Model file for the job. Use its own axes, mm. Give positions to 0.01 mm unless a question says otherwise; leave off trailing zeros. Order: outer loops, then holes, each group sorted by start corner. A loop starts at its lowest first (then second) coordinate and runs counter-clockwise, first axis right, second up. Notation, with made-up numbers: (-31.5, -11.75) -> (23.5, -11.75) arc R10 ccw to (23.5, -5.75) -> close; hole circle Ø10 at (19.5, 1.25). An arc over 180 degrees is marked (long way). Use CSV: the item, a comma, the result in double quotes. Start each with the question number.
1. Cut at C-C on z = -2. List the corners of the cut face in (x, y).
2. Cut at D-D on x = 61. List the corners of the cut face in (y, z) (3 decimals).
3. Cut at A-A on y = -50.8. List the corners of the cut face in (x, z) (3 decimals).
4. Wall check: line 1 (Y direction, x = 0, z = -1); line 2 (X direction, y = -52, z = -0.5); line 3 (X direction, y = -48.5, z = 0.25). Give the ranges that are in metal, low to high. Write a range as from..to.
5. Drop flat-ended pins along their axis: pin 1 (1 mm diameter, centred on y = -60.5, z = -1.5, fed in from -X); pin 2 (14.5 mm diameter, centred on x = 0, y = -50.8, fed in from -Z) (3 decimals); pin 3 (2 mm diameter, centred on x = 78.5, z = 2, fed in from -Y). Give the stop position or say it passes through.
6. Cut at B-B on x = 0. List the corners of the cut face in (y, z) (3 decimals), then the cut area to 3 significant figures.
```python
from build123d import *

# Parameters (mm, degrees)
BOSS_EXTRUDE1_DEPTH = 3.175
SKETCH2_R           = 6.35
CUT_EXTRUDE1_DEPTH  = 136.152108752


with BuildPart() as part:
    # Sketch1 → Boss-Extrude1 (new, symmetric)
    with BuildSketch(Plane.XY):
        Polygon((-101.6, 0), (-12.7, -88.9), (12.7, -88.9), (101.6, 0), align=None)
    extrude(amount=BOSS_EXTRUDE1_DEPTH, both=True)

    # Sketch2 → Cut-Extrude1 (cut, through all)
    with BuildSketch(Plane.XY.offset(3.175)):
        with Locations((0, -50.8)):
            Circle(SKETCH2_R)
    extrude(amount=-CUT_EXTRUDE1_DEPTH, mode=Mode.SUBTRACT)


solid = part.part
```
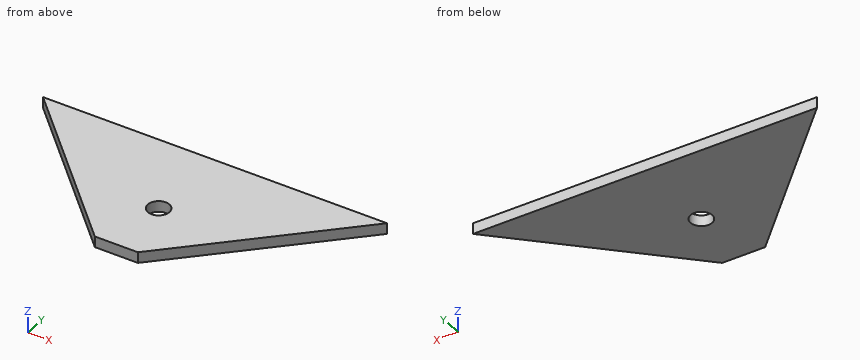
Verdict:
1,outline,"(-101.6, 0) -> (-12.7, -88.9) -> (12.7, -88.9) -> (101.6, 0) -> close; hole circle Ø12.7 at (0, -50.8)"
2,outline,"(-40.6, -3.175) -> (0, -3.175) -> (0, 3.175) -> (-40.6, 3.175) -> close"
3,outline,"(-50.8, -3.175) -> (-6.35, -3.175) -> (-6.35, 3.175) -> (-50.8, 3.175) -> close; (6.35, -3.175) -> (50.8, -3.175) -> (50.8, 3.175) -> (6.35, 3.175) -> close"
4,line 1,"-88.9..-57.15, -44.45..0"
4,line 2,"-49.6..-6.24, 6.24..49.6"
4,line 3,"-53.1..-5.92, 5.92..53.1"
5,pin 1,"x = -41.6"
5,pin 2,"z = -3.175"
5,pin 3,"y = -24.1"
6,outline,"(-88.9, -3.175) -> (-57.15, -3.175) -> (-57.15, 3.175) -> (-88.9, 3.175) -> close; (-44.45, -3.175) -> (0, -3.175) -> (0, 3.175) -> (-44.45, 3.175) -> close"
6,area,"484 mm^2"
